Geometry: final body of the model. Coordinates: model frame, mm. Give positions to 0.01 mm unless a question says otherwise; leave off trailing zeros. Write each loop counter-clockwise with the first axis right and the second up, starting at its lowest first coordinate (ties: lowest second). Pieces come first, ordered by that corner, then holes.
from build123d import *

# Parameters (mm, degrees)
ESQUISSE1_W             = 430
ESQUISSE1_H             = 450
BOSS_EXTRU_1_DEPTH      = 22
ENL_V_START             = -22
ESQUISSE2_W             = 250
ESQUISSE2_H             = 275
ENL_V_MAT_EXTRU_1_DEPTH = 1
ESQUISSE3_R             = 3
ENL_V_MAT_EXTRU_2_DEPTH = 623.803339747


with BuildPart() as part:
    # Esquisse1 → Boss.-Extru.1 (new body)
    with BuildSketch(Plane.XY):
        with Locations((215, 225)):
            Rectangle(ESQUISSE1_W, ESQUISSE1_H)
    extrude(amount=BOSS_EXTRU_1_DEPTH)

    # Esquisse2 → Enlèv. mat.-Extru.1 (cut)
    with BuildSketch(Plane.XY.offset(22).offset(ENL_V_START)):
        with Locations((235, 252.5)):
            Rectangle(ESQUISSE2_W, ESQUISSE2_H)
    extrude(amount=ENL_V_MAT_EXTRU_1_DEPTH, mode=Mode.SUBTRACT)

    # Esquisse3 → Enlèv. mat.-Extru.2 (cut, through all)
    with BuildSketch(Plane(origin=(0, 0, 0), x_dir=(-1, 0, 0), z_dir=(0, 0, -1))):
        with Locations((-385, 277.5)):
            Circle(ESQUISSE3_R)
        with Locations(Location((-335, 277.5, 0), (0, 0, 180))):
            Circle(ESQUISSE3_R)
        with Locations((-135, 77.5)):
            Circle(ESQUISSE3_R)
        with Locations(Location((-85, 77.5, 0), (0, 0, 180))):
            Circle(ESQUISSE3_R)
        with Locations(Location((-185, 77.5, 0), (0, 0, 180))):
            Circle(ESQUISSE3_R)
        with Locations((-285, 77.5)):
            Circle(ESQUISSE3_R)
        with Locations((-285, 277.5)):
            Circle(ESQUISSE3_R)
        with Locations(Location((-235, 277.5, 0), (0, 0, 180))):
            Circle(ESQUISSE3_R)
        with Locations(Location((-185, 277.5, 0), (0, 0, 180))):
            Circle(ESQUISSE3_R)
        with Locations(Location((-235, 77.5, 0), (0, 0, 180))):
            Circle(ESQUISSE3_R)
        with Locations((-385, 77.5)):
            Circle(ESQUISSE3_R)
        with Locations(Location((-335, 77.5, 0), (0, 0, 180))):
            Circle(ESQUISSE3_R)
        with Locations((-135, 277.5)):
            Circle(ESQUISSE3_R)
        with Locations(Location((-85, 277.5, 0), (0, 0, 180))):
            Circle(ESQUISSE3_R)
        with Locations((-85, 327.5)):
            Circle(ESQUISSE3_R)
        with Locations(Location((-135, 327.5, 0), (0, 0, 180))):
            Circle(ESQUISSE3_R)
        with Locations((-135, 377.5)):
            Circle(ESQUISSE3_R)
        with Locations(Location((-85, 377.5, 0), (0, 0, 180))):
            Circle(ESQUISSE3_R)
        with Locations(Location((-185, 377.5, 0), (0, 0, 180))):
            Circle(ESQUISSE3_R)
        with Locations((-185, 327.5)):
            Circle(ESQUISSE3_R)
        with Locations((-235, 327.5)):
            Circle(ESQUISSE3_R)
        with Locations(Location((-285, 327.5, 0), (0, 0, 180))):
            Circle(ESQUISSE3_R)
        with Locations((-285, 377.5)):
            Circle(ESQUISSE3_R)
        with Locations(Location((-235, 377.5, 0), (0, 0, 180))):
            Circle(ESQUISSE3_R)
        with Locations((-385, 377.5)):
            Circle(ESQUISSE3_R)
        with Locations(Location((-335, 377.5, 0), (0, 0, 180))):
            Circle(ESQUISSE3_R)
        with Locations((-335, 327.5)):
            Circle(ESQUISSE3_R)
        with Locations(Location((-385, 327.5, 0), (0, 0, 180))):
            Circle(ESQUISSE3_R)
        with Locations((-385, 177.5)):
            Circle(ESQUISSE3_R)
        with Locations(Location((-335, 177.5, 0), (0, 0, 180))):
            Circle(ESQUISSE3_R)
        with Locations((-335, 127.5)):
            Circle(ESQUISSE3_R)
        with Locations(Location((-385, 127.5, 0), (0, 0, 180))):
            Circle(ESQUISSE3_R)
        with Locations((-235, 127.5)):
            Circle(ESQUISSE3_R)
        with Locations(Location((-285, 127.5, 0), (0, 0, 180))):
            Circle(ESQUISSE3_R)
        with Locations((-285, 177.5)):
            Circle(ESQUISSE3_R)
        with Locations(Location((-235, 177.5, 0), (0, 0, 180))):
            Circle(ESQUISSE3_R)
        with Locations(Location((-185, 177.5, 0), (0, 0, 180))):
            Circle(ESQUISSE3_R)
        with Locations((-185, 127.5)):
            Circle(ESQUISSE3_R)
        with Locations((-85, 127.5)):
            Circle(ESQUISSE3_R)
        with Locations(Location((-135, 127.5, 0), (0, 0, 180))):
            Circle(ESQUISSE3_R)
        with Locations((-135, 177.5)):
            Circle(ESQUISSE3_R)
        with Locations(Location((-85, 177.5, 0), (0, 0, 180))):
            Circle(ESQUISSE3_R)
        with Locations((-85, 227.5)):
            Circle(ESQUISSE3_R)
        with Locations(Location((-135, 227.5, 0), (0, 0, 180))):
            Circle(ESQUISSE3_R)
        with Locations((-185, 227.5)):
            Circle(ESQUISSE3_R)
        with Locations((-235, 227.5)):
            Circle(ESQUISSE3_R)
        with Locations(Location((-285, 227.5, 0), (0, 0, 180))):
            Circle(ESQUISSE3_R)
        with Locations((-335, 227.5)):
            Circle(ESQUISSE3_R)
        with Locations(Location((-385, 227.5, 0), (0, 0, 180))):
            Circle(ESQUISSE3_R)
        with Locations((-335, 427.5)):
            Circle(ESQUISSE3_R)
        with Locations(Location((-385, 427.5, 0), (0, 0, 180))):
            Circle(ESQUISSE3_R)
        with Locations((-235, 427.5)):
            Circle(ESQUISSE3_R)
        with Locations(Location((-285, 427.5, 0), (0, 0, 180))):
            Circle(ESQUISSE3_R)
        with Locations((-185, 427.5)):
            Circle(ESQUISSE3_R)
        with Locations((-85, 427.5)):
            Circle(ESQUISSE3_R)
        with Locations(Location((-135, 427.5, 0), (0, 0, 180))):
            Circle(ESQUISSE3_R)
    extrude(amount=-ENL_V_MAT_EXTRU_2_DEPTH, mode=Mode.SUBTRACT)


solid = part.part
Q1. Section A-A on y = 368.5. Output: boundary loops of the cut face in (x, z), plus the area to 3 significant figures.
Filled sheet:
outline: (0, 0) - (110, 0) - (110, 1) - (360, 1) - (360, 0) - (430, 0) - (430, 22) - (0, 22) - close
area: 9,210 mm2
Q2. Section B-B on x = 309. Output: boundary loops of the cut face in (y, z).
Filled sheet:
outline: (0, 0) - (115, 0) - (115, 1) - (390, 1) - (390, 0) - (450, 0) - (450, 22) - (0, 22) - close
Q3. Pull-direction query (X, two-part tool) for faces 1 (the flat face through (212, 0, 11)), 2 (the flat face through (0, 222, 11)), 3 (the flat face through (233, 254, 1)); classes: released by +X, released by -X, zero draft, split by the parting line, or undercut.
Filled sheet:
face 1: zero draft
face 2: released by -X
face 3: undercut
Q4. Pin query (flat end, axial travel): P1, Ø4, axis at x = 182.5, y = 127, coming from the -Z side; P2, Ø5.5, axis at x = 285, y = 277.5, coming from the +Z side. Return the tip coordinate at first contact, or that it passes through.
Filled sheet:
P1: stops at z = 1
P2: passes through
Q5. Ray query, line 1 along Z through (x, y) = (223, 183). Return the intervals inside material, ascending.
Filled sheet:
line 1: z = 1 to 22
